Geometry check sheet. Reference: the model listing, model coordinates, mm. Face numbers are marked on the shaded views. A direction names the side the tool comes from. Give positions to 0.01 mm unless a question says otherwise; leave off trailing zeros. Order: outer loops, then holes, each group sorted by start corner. A loop starts at its lowest first (then second) coordinate and runs counter-clockwise, first axis right, second up. Notation, with made-up numbers: M -11.75,-28 L 25.25,-28 A21 cw 25.25,9 Z; hole C 84,5.5 d2. An arc over 180 degrees is marked long. Answer as CSV lines item,"result". Start each with the question number.
```python
from build123d import *

# Parameters (mm, degrees)
SKETCH_R      = 40
SKETCH_R_2    = 25
PAD_DEPTH     = 40
PAD001_DEPTH  = 500
SKETCH002_R   = 40
SKETCH002_R_2 = 25
PAD002_DEPTH  = 40
PAD003_DEPTH  = 5
PAD004_DEPTH  = 5
PAD005_DEPTH  = 5
PAD006_DEPTH  = 5


with BuildPart() as part:
    # Sketch → Pad (new body, symmetric)
    with BuildSketch(Plane.XZ):
        Circle(SKETCH_R)
        Circle(SKETCH_R_2, mode=Mode.SUBTRACT)
    extrude(amount=PAD_DEPTH, both=True)

    # Sketch001 → Pad001 (join)
    with BuildSketch(Plane.YZ):
        Polygon((-30, 50), (-30, 40), (-40, 40), (-40, 30), (-20, 30), (-20, 50), align=None)
        Polygon((30, 50), (30, 40), (40, 40), (40, 30), (20, 30), (20, 50), align=None)
        Polygon((-30, -50), (-30, -40), (-40, -40), (-40, -30), (-20, -30), (-20, -50), align=None)
        Polygon((30, -50), (30, -40), (40, -40), (40, -30), (20, -30), (20, -50), align=None)
    extrude(amount=PAD001_DEPTH)

    # Sketch002 → Pad002 (join, symmetric)
    with BuildSketch(Plane(origin=(500, 0, 0), x_dir=(1, 0, 0), z_dir=(0, -1, 0))):
        Circle(SKETCH002_R)
        Circle(SKETCH002_R_2, mode=Mode.SUBTRACT)
    extrude(amount=PAD002_DEPTH, both=True)

    # Sketch004 → Pad003 (join, symmetric)
    with BuildSketch(Plane.XZ.offset(-30)):
        Polygon((80, -30), (140, 30), (150, 30), (90, -30), align=None)
        Polygon((450, -30), (430, -30), (380, 30), (400, 30), align=None)
        Polygon((180.003479, 30.370306), (240.003479, -29.629694), (250, -29.629694), (190, 30.370306), align=None)
        Polygon((358.794617, 29.393638), (340, 29.393638), (280, -30.606362), (298.794617, -30.606362), align=None)
    extrude(amount=PAD003_DEPTH, both=True)

    # Sketch003 → Pad004 (join, symmetric)
    with BuildSketch(Plane.XZ.offset(30)):
        Polygon((80, -30), (140, 30), (150, 30), (90, -30), align=None)
        Polygon((450, -30), (430, -30), (380, 30), (400, 30), align=None)
        Polygon((180, 30), (240, -30), (250, -30), (190, 30), align=None)
        Polygon((357.920776, 30), (340, 30), (280, -30), (300, -30), align=None)
    extrude(amount=PAD004_DEPTH, both=True)

    # Sketch006 → Pad005 (join, symmetric)
    with BuildSketch(Plane.XY.offset(-40)):
        Polygon((230, 20), (190, -20), (180, -20), (220, 20), align=None)
        Polygon((160, -20), (120, 20), (110, 20), (150, -20), align=None)
        Polygon((90, 20), (50, -20), (40, -20), (80, 20), align=None)
        Polygon((270, 20), (310, -20), (320, -20), (280, 20), align=None)
        Polygon((340, -20), (380, 20), (390, 20), (350, -20), align=None)
        Polygon((410, 20), (450, -20), (460, -20), (420, 20), align=None)
    extrude(amount=PAD005_DEPTH, both=True)

    # Sketch005 → Pad006 (join, symmetric)
    with BuildSketch(Plane.XY.offset(40)):
        Polygon((230, 20), (190, -20), (180, -20), (220, 20), align=None)
        Polygon((160, -20), (120, 20), (110, 20), (150, -20), align=None)
        Polygon((90, 20), (50, -20), (40, -20), (80, 20), align=None)
        Polygon((270, 20), (310, -20), (320, -20), (280, 20), align=None)
        Polygon((340, -20), (380, 20), (390, 20), (350, -20), align=None)
        Polygon((410, 20), (450, -20), (460, -20), (420, 20), align=None)
    extrude(amount=PAD006_DEPTH, both=True)


solid = part.part
```
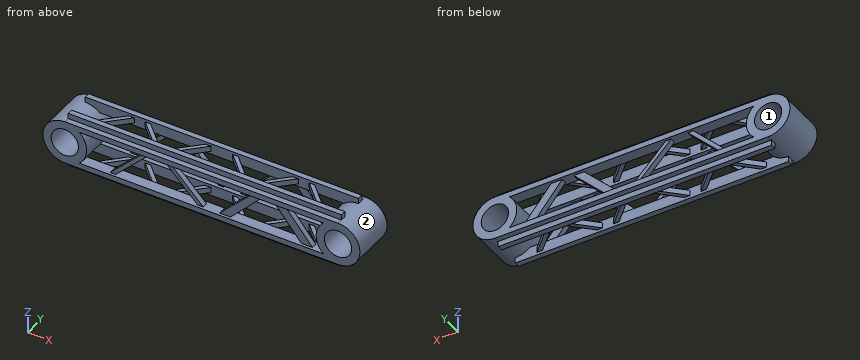
Item 1: Section check A-A on x = 327. Give the number of separate pieces and of enclosed holes in the cut face, then the cut area to 3 significant figures.
Item 2: Depth check by flat-ended pin: pin 1 Ø12 at (x, z) = (325, -5.5) entering from -Y; pin 2 Ø8 at (x, y) = (178.5, -34.5) entering from -Z; pin 3 Ø11 at (y, z) = (27.5, 46.5) entering from +X. Enter the tip coordinate at first touch or a pass-through.
Item 3: Section check C-C on x = 8. Record the boundary of the cut face in (y, z), then the cut area to 3 significant figures.
Item 4: Access from +Z, -Z, +X, -X, +Y, -Y to the whole of each face (thin tool, end or side, straight path). Record for the marked faces 1 and 2.
Item 5: Scan lines: line 1 along Y through (x, z) = (407.5, 7.5); line 2 along Z through (x, y) = (0, -6); line 3 along Y through (x, z) = (239, -41.5). Record each from-to range of solid material in increasing order.
Numbers:
1,separate pieces,"6"
1,enclosed holes,"0"
1,area,"1,580 mm2"
2,pin 1,"y = -35"
2,pin 2,"z = -40"
2,pin 3,"x = 500"
3,outline,"M -40,-40 L -30,-40 L -30,-50 L -20,-50 L -20,-39.19 L 20,-39.19 L 20,-50 L 30,-50 L 30,-40 L 40,-40 L 40,-23.69 L -40,-23.69 Z; M -40,23.69 L 40,23.69 L 40,40 L 30,40 L 30,50 L 20,50 L 20,39.19 L -20,39.19 L -20,50 L -30,50 L -30,40 L -40,40 Z"
3,area,"2,950 mm2"
4,face 1,"+Y, -Y"
4,face 2,"none"
5,line 1,"-35 to -25, 25 to 35"
5,line 2,"-40 to -25, 25 to 40"
5,line 3,"-30 to -20, 20 to 30"
